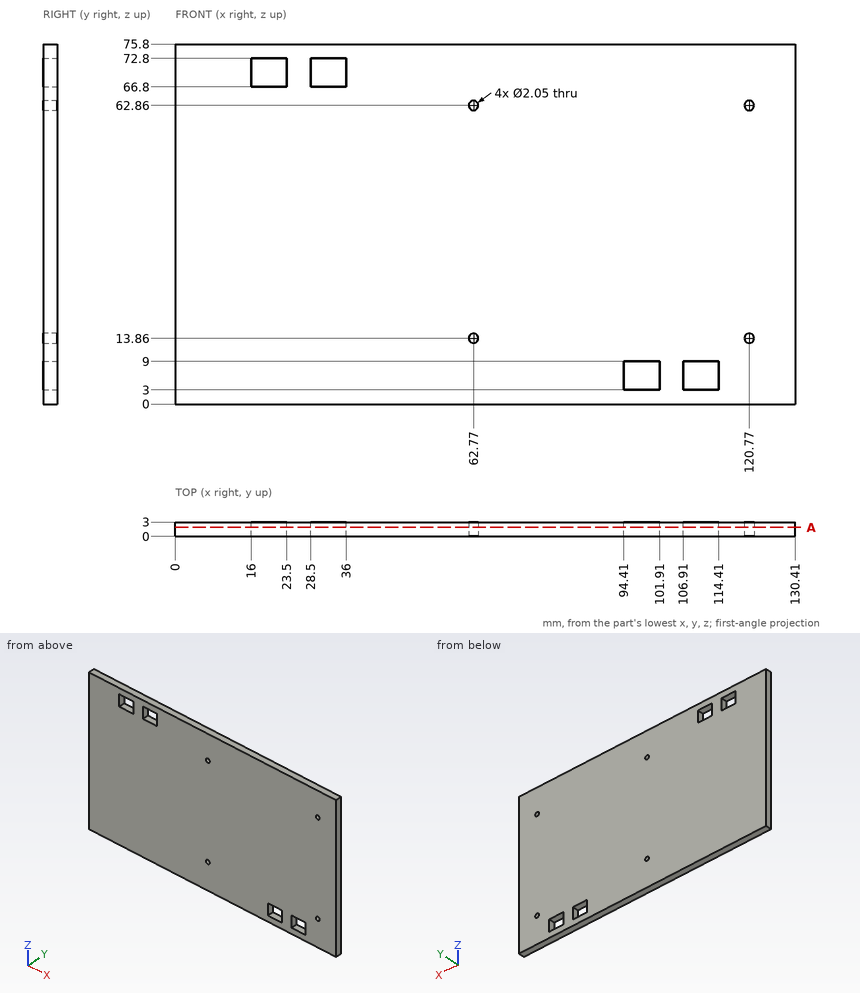
Can you work these out from the drawing? Everything is in mm from the part's minimum corner. Round coordinates to 2 decimals unless told otherwise and drop trailing zeros. One line per question, with ' | ' between items.
1) I want a section at A-A, the plane y = 1.9. State how many separate pieces and enclosed holes the cut face has, then the cut area to 3 significant figures.
Working result:
separate pieces: 1 | enclosed holes: 8 | area: 9,690 mm²
2) I need wall thicknesses on line 1 along X through (y, z) = (1.4, 13.86) (3 decimals); line 2 along X through (y, z) = (1.15, 68); line 3 along Z through (x, y) = (19, 1.1). Which ranges of each line are inside material? Lowest first, please.
Working result:
line 1: 0 to 61.745, 63.795 to 119.745, 121.795 to 130.41 | line 2: 0 to 16, 23.5 to 28.5, 36 to 130.41 | line 3: 0 to 66.8, 72.8 to 75.8
3) For pin 1 Ø1.2 at (x, z) = (120.77, 13.86) entering from -Y, with a flat end and sliding along its axis, tell me the tip position at first contact or that it passes through.
Working result:
pin 1: through
